Geometry: final body of the model. Coordinates: model frame, mm. A direction names the side the tool comes from. Round coordinates to 2 decimals unless told otherwise and drop trailing zeros. Loops run counter-clockwise (first coordinate to the right, second up) from the corner with the lowest first, then second, coordinate; pieces in that order, holes last. Notation, with made-up numbers: (-16.75, 6) - (32.25, 6) arc R26 cw to (32.25, 24) - close; hole circle Ø11 at (31, 42.25). An arc over 180 degrees is marked (long way). Answer in a Markdown table with one row per item. Add a question column.
from build123d import *

# Parameters (mm, degrees)
SKETCH1_R           = 4.95
SKETCH1_R_2         = 1
SKETCH1_R_3         = 0.75
BOSS_EXTRUDE1_DEPTH = 11.8
SKETCH1_3_R         = 0.75
BOSS_EXTRUDE2_DEPTH = 18.1
CUT_EXTRUDE1_START  = 11.8
SKETCH1_5_R         = 1
CUT_EXTRUDE1_DEPTH  = 2


with BuildPart() as part:
    # Sketch1 → Boss-Extrude1 (new body)
    # profile 1 of 5: a face of its own
    with BuildSketch(Plane.XY):
        Circle(SKETCH1_R)
        with Locations((-3.5, 0)):
            Circle(SKETCH1_R_2, mode=Mode.SUBTRACT)
        with Locations((0, -3.5)):
            Circle(SKETCH1_R_2, mode=Mode.SUBTRACT)
        with Locations((3.5, 0)):
            Circle(SKETCH1_R_2, mode=Mode.SUBTRACT)
        with Locations((0, 3.5)):
            Circle(SKETCH1_R_2, mode=Mode.SUBTRACT)
        Circle(SKETCH1_R_3, mode=Mode.SUBTRACT)
    # profile 2 of 5: a face of its own
    with BuildSketch(Plane.XY):
        with Locations((-3.5, 0)):
            Circle(SKETCH1_R_2)
    # profile 3 of 5: a face of its own
    with BuildSketch(Plane.XY):
        with Locations((0, 3.5)):
            Circle(SKETCH1_R_2)
    # profile 4 of 5: a face of its own
    with BuildSketch(Plane.XY):
        with Locations((3.5, 0)):
            Circle(SKETCH1_R_2)
    # profile 5 of 5: a face of its own
    with BuildSketch(Plane.XY):
        with Locations((0, -3.5)):
            Circle(SKETCH1_R_2)
    extrude(amount=BOSS_EXTRUDE1_DEPTH)

    # Sketch1<3> → Boss-Extrude2 (add)
    with BuildSketch(Plane.XY):
        with Locations(Location((0, 0, 0), (0, 0, 180))):
            Circle(SKETCH1_3_R)
    extrude(amount=BOSS_EXTRUDE2_DEPTH)

    # Sketch1<5> → Cut-Extrude1 (cut)
    with BuildSketch(Plane.XY.offset(CUT_EXTRUDE1_START)):
        with Locations((0, 3.5)):
            Circle(SKETCH1_5_R)
        with Locations((-3.5, 0)):
            Circle(SKETCH1_5_R)
        with Locations((3.5, 0)):
            Circle(SKETCH1_5_R)
        with Locations((0, -3.5)):
            Circle(SKETCH1_5_R)
    extrude(amount=-CUT_EXTRUDE1_DEPTH, mode=Mode.SUBTRACT)


solid = part.part
1) Section A-A, the plane y = 0. Return the cut outline in (x, z).
2) Pull-direction query (Y, two-part tool) for faces 3 (the cylindrical face through (-4.5, 0, 10.8)), 4 (the cylindrical face through (4.72, 1.49, 5.82)), 5 (the flat face through (0, 0, 0)); classes: pulls with the +Y half, pulls with the -Y half, needs draft (parallel to the pull), parting line crosses it, or undercut.
3) Section C-C, the plane z = 9.5. Return the cut outline in (x, y), and give its area (3 significant figures).
4) Contact query for flat-ended pins moving along their axis: pin 1 Ø3 at (x, y) = (0, -3.5) entering from +Z; pin 2 Ø5 at (y, z) = (0.5, 14.5) entering from +X; pin 3 Ø1 at (x, z) = (-2, 6) entering from -Y. Output: stop coordinate, or through.
5) Section D-D, the plane y = 3.5. Return the cut outline in (x, z).
6) Reachability of faces 1 (the cylindrical face through (0.954, -3.2, 10.814)), 2 (the flat face through (0, 0, 18.1)) from +Z, -Z, +X, -X, +Y, -Y: full face, straight path, thin tool, end or side. Return the list, or none.
7) Material intervals for line 1 along Y through (x, z) = (0, 11.35); line 2 along Z through (x, y) = (2.5, -3.75); line 3 along Z through (x, y) = (-3.5, -0.5), sorted ascending. Write a range as from..to.
Evaluation:
| question | item | result |
|---|---|---|
| 1 | outline | (-4.95, 0) - (4.95, 0) - (4.95, 11.8) - (4.5, 11.8) - (4.5, 9.8) - (2.5, 9.8) - (2.5, 11.8) - (0.75, 11.8) - (0.75, 18.1) - (-0.75, 18.1) - (-0.75, 11.8) - (-2.5, 11.8) - (-2.5, 9.8) - (-4.5, 9.8) - (-4.5, 11.8) - (-4.95, 11.8) - close |
| 2 | face 3 | undercut |
| 2 | face 4 | parting line crosses it |
| 2 | face 5 | needs draft |
| 3 | outline | circle Ø9.9 at (0, 0) |
| 3 | area | 77.0 mm² |
| 4 | pin 1 | stops at z = 11.8 |
| 4 | pin 2 | stops at x = 0.75 |
| 4 | pin 3 | stops at y = -4.72 |
| 5 | outline | (-3.5, 0) - (3.5, 0) - (3.5, 11.8) - (1, 11.8) - (1, 9.8) - (-1, 9.8) - (-1, 11.8) - (-3.5, 11.8) - close |
| 6 | face 1 | +Z |
| 6 | face 2 | +Z, +X, -X, +Y, -Y |
| 7 | line 1 | y = -4.95..-4.5, -2.5..2.5, 4.5..4.95 |
| 7 | line 2 | z = 0..11.8 |
| 7 | line 3 | z = 0..9.8 |
